```python
from build123d import *

# Parameters (mm, degrees)
F0_W     = 15
F0_H     = 15
F0_R     = 6.625
F1_DEPTH = 2.4
F2_W     = 15
F2_H     = 15
F3_DEPTH = 1.7
F4_D     = 5.25


with BuildPart() as f1:
    # F0 (on Top) → F1 (new body)
    with BuildSketch(Plane.XY):
        Rectangle(F0_W, F0_H)
        Circle(F0_R, mode=Mode.SUBTRACT)
    extrude(amount=F1_DEPTH)

    # F2 (on face) → F3 (join)
    with BuildSketch(Plane.XY.offset(2.4)):
        Rectangle(F2_W, F2_H)
    extrude(amount=F3_DEPTH)

    # F4 (through all)
    with Locations(Plane(origin=(0, 0, 0), x_dir=(1, 0, 0), z_dir=(0, 0, -1))):
        with Locations((0, 0)):
            Hole(F4_D / 2)


solid = f1.part
```
Design review of the part built by this model. Coordinates are the model's own, in mm. A direction names the side the tool comes from. Coordinates: 2 decimals unless noted, no trailing zeros. Order: outer loops, then holes, each group sorted by start corner. A loop starts at its lowest first (then second) coordinate and runs counter-clockwise, first axis right, second up.
1) Take a section at D-D, the plane y = -3.75. Give the boundary of the cut face in (x, z), and give its area (3 significant figures).
2) Wall thickness on line 1 along Y through (x, z) = (0, 1.35) (3 decimals); line 2 along Z through (x, y) = (-3.5, 4); line 3 along Y through (x, z) = (0, 3.1) (3 decimals): over which ranges is each line inside the solid? List them lowest first.
3) For faces 5 (the flat face through (-7.5, 0, 2)), 6 (the flat face through (3, 0, 2.4)), list the 3-axis set-ups (+Z, -Z, +X, -X, +Y, -Y) from which the entire face can be reached by the end or side of a thin tool; tool diameter is ignored.
4) Take a section at C-C, the plane z = 2.8. Give the boundary of the cut face in (x, y) (3 decimals).
5) Take a section at A-A, the plane y = 0. Give the boundary of the cut face in (x, z) (3 decimals), and give its area (3 significant figures).
6) Mouldability with a two-part tool opening along Y and no side actions: class faces 1 (the cylindrical face through (3.562, 5.586, 1.183)), 2 (the flat face through (0, 7.5, 2)), 3 (the flat face through (-3, 0, 4.1)), 4 (the cylindrical face through (-2.5, -0.8, 3.3)) as +Y half, -Y half, draft (parallel to the pull), parting line (faces both ways), or undercut.
Returned:
1. outline: (-7.5, 0) - (-5.46, 0) - (-5.46, 2.4) - (5.46, 2.4) - (5.46, 0) - (7.5, 0) - (7.5, 4.1) - (-7.5, 4.1) - close
1. area: 35.3 mm2
2. line 1: y = -7.5 to -6.625, 6.625 to 7.5
2. line 2: z = 2.4 to 4.1
2. line 3: y = -7.5 to -2.625, 2.625 to 7.5
3. face 5: +Z, -Z, -X, +Y, -Y
3. face 6: -Z
4. outline: (-7.5, -7.5) - (7.5, -7.5) - (7.5, 7.5) - (-7.5, 7.5) - close; hole circle Ø5.25 at (0, 0)
5. outline: (-7.5, 0) - (-6.625, 0) - (-6.625, 2.4) - (-2.625, 2.4) - (-2.625, 4.1) - (-7.5, 4.1) - close; (2.625, 2.4) - (6.625, 2.4) - (6.625, 0) - (7.5, 0) - (7.5, 4.1) - (2.625, 4.1) - close
5. area: 20.8 mm2
6. face 1: undercut
6. face 2: +Y half
6. face 3: draft
6. face 4: undercut
